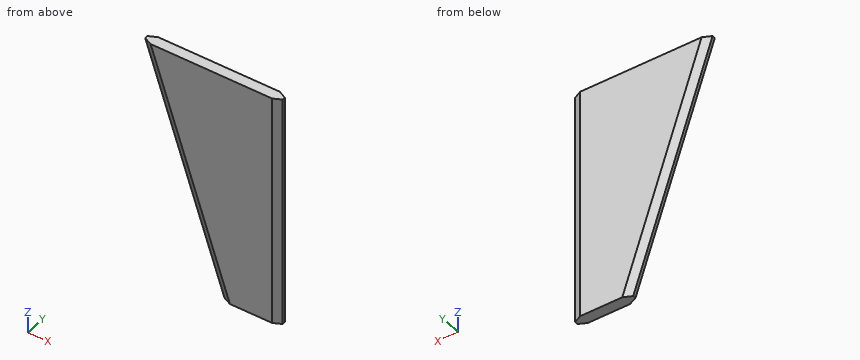
Autodesk Inventor part; units mm, degrees
ref_plane "Work Plane1" through (0, 14, 0) normal (0, 1, 0) x (1, 0, 0)
ref_plane "YZ Plane" through (0, 0, 0) normal (1, 0, 0) x (0, 1, 0)
ref_plane "XZ Plane" through (0, 0, 0) normal (0, 1, 0) x (-1, 0, 0)
sketch "Sketch1" plane through (0, 0, 0) normal (0, 1, 0) x (-1, 0, 0)
  line L0 (0, 0) -> (355, 0)
  line L1 (355, 0) -> (355, -600)
  line L2 (355, -600) -> (0, -600)
  line L3 (0, -600) -> (0, 0)
  dimension "d0" = 600
  dimension "d1" = 355
extrude "Extrusion1" add sketch "Sketch1" along normal blind 28
sketch "Sketch2" plane through (0, 28, 0) normal (0, 1, 0) x (1, 0, 0)
  line L0 (-355, 600) -> (-355, 0)
  line L1 (0, 600) -> (-355, 600)
  line L2 (0, 600) -> (-355, 600)
  line L3 (-355, 600) -> (-355, 0)
  line L4 (-355, 0) -> (0, 0)
  line L5 (0, 0) -> (0, 600)
  line L6 (-355, 0) -> (-150, 600)
  point P0 (-150, 600)
  dimension "d7" = 150
  dimension "d8" = 0
extrude "Extrusion2" cut sketch "Sketch2" against normal blind 200 contours L1 L6 L0
ref_plane "Work Plane1" through (0, 14, 0) normal (0, 1, 0) x (1, 0, 0)
chamfer "Chamfer1" distance 20 distance2 10 1 edges at (0, 28, -300) measured on face at (-168.3333, 28, -200)
chamfer "Chamfer2" distance 10 distance2 20 1 edges at (0, 0, -300) measured on face at (0, 6, -200)
chamfer "Chamfer3" distance 20 distance2 10 1 edges at (-252.5, 28, -300) measured on face at (-175, 28, -200)
chamfer "Chamfer4" distance 20 distance2 10 1 edges at (-252.5, 0, -300) measured on face at (-175, 0, -200)
properties part number "Foam_wing_V2"
Can you work these out from the model? Positions are in its coordinate system, mm. Coordinates: 2 decimals unless noted, no trailing zeros. Loops run counter-clockwise (first coordinate to the right, second up) from the corner with the lowest first, then second, coordinate; pieces in that order, holes last. Notation, with made-up numbers: (48.25, 51) -> (86.25, 51) arc R12 cw to (86.25, 70) -> close; hole circle Ø11 at (7, 58). An arc over 180 degrees is marked (long way). Put each result on its own line as item: value. Start each with the question number.
Q1. If I drill on line 1 (X direction, y = 5, z = -72); line 2 (X direction, y = 26.25, z = -494.5); line 3 (Y direction, x = -204, z = -410.5), over which ranges is the centre line in solid material (lowest first)? Write a range as [from, to].
Q2. I want a section at C-C (y = 23.5). Write out the boundary of the cut face in (x, z).
Q3. I want a section at D-D (z = -81.5). Write out the boundary of the cut face in (x, y), plus the area to 3 significant figures.
Q4. I want a section at B-B (x = -285.5). Write out the boundary of the cut face in (y, z), plus the area to 3 significant figures.
Q5. I want a section at A-A (z = -334.5). Write out the boundary of the cut face in (x, y), plus the area to 3 significant figures.
Q6. I'm going to push flat-ended pins straight in: P1, Ø12, axis at y = 23.5, z = -66, coming from the -X side; P2, Ø2, axis at y = 21.5, z = -489.5, coming from the -X side; P3, Ø4, axis at y = 4.5, z = -388, coming from the -X side. Where does each tip first touch, or does it pass through?
Taken from the geometry:
1. line 1: x = [-319.83, -10]
1. line 2: x = [-168.61, -16.5]
1. line 3: y = [4.92, 23.08]
2. outline: (-343.38, 0) -> (-138.38, -600) -> (-11, -600) -> (-11, 0) -> close
3. outline: (-327.15, 10) -> (-306.02, 0) -> (-20, 0) -> (0, 10) -> (0, 18) -> (-20, 28) -> (-306.02, 28) -> (-327.15, 18) -> close
3. area: 8,750 mm2
4. outline: (0, -141.56) -> (10, -203.41) -> (18, -203.41) -> (28, -141.56) -> (28, 0) -> (0, 0) -> close
4. area: 5,080 mm2
5. outline: (-240.71, 10) -> (-219.58, 0) -> (-20, 0) -> (0, 10) -> (0, 18) -> (-20, 28) -> (-219.58, 28) -> (-240.71, 18) -> close
5. area: 6,330 mm2
6. P1: stops at x = -333.27
6. P2: stops at x = -182.5
6. P3: stops at x = -215.09
